Source: CAD feature listing. Evaluate the final solid. Frame: model axes, mm. A direction names the side the tool comes from. Give positions to 0.01 mm unless a question says otherwise; leave off trailing zeros. Write each loop counter-clockwise with the first axis right and the second up, starting at its lowest first coordinate (ties: lowest second). Pieces come first, ordered by that corner, then holes. Notation, with made-up numbers: M 35,-38 L 68,-38 A20 cw 68,-23 Z; hole C -25,24 d11. An arc over 180 degrees is marked long. Use CSV: the item, a comma, the result in double quotes. Start each with the question number.
from build123d import *

# Parameters (mm, degrees)
SKETCH_1_W               = 3
SKETCH_1_H               = 8
SKETCH_2_R               = 7.25
CUT_EXTRUDE_1_DEPTH      = 1
EXTRUDE_START            = 10
EXTRUDE_1_DEPTH          = 10
CUT_EXTRUDE_2_DEPTH      = 48.607194834
CUT_EXTRUDE_2_DEPTH_BACK = 48.607194834
SKETCH_4_R               = 1.55


with BuildPart() as part:
    # 草图1 → 旋转1 (revolve)
    with BuildSketch(Plane.XY, mode=Mode.PRIVATE) as revolve_1_sk:
        Polygon((0, 42), (0, 39.9), (7.85, 39.9), (15.85, 39.9), (15.85, 42), align=None)
        Polygon((0, 39.9), (0, 8), (3, 8), (7.85, 8), (7.85, 39.9), align=None)
        with Locations((1.5, 4)):
            Rectangle(SKETCH_1_W, SKETCH_1_H)
    revolve(revolve_1_sk.sketch.rotate(Axis((0, 0, 0), (0, 1, 0)), 90), axis=Axis((0, 0, 0), (0, 1, 0)))

    # 草图2 → 切除-拉伸1 (cut)
    with BuildSketch(Plane(origin=(0, 42, 0), x_dir=(1, 0, 0), z_dir=(0, 1, 0))):
        with Locations(Location((0, 0, 0), (0, 0, 270))):
            Circle(SKETCH_2_R)
    extrude(amount=-CUT_EXTRUDE_1_DEPTH, mode=Mode.SUBTRACT)

    # 草图3 → 凸台-拉伸1 (add)
    with BuildSketch(Plane(origin=(0, 41, 0), x_dir=(1, 0, 0), z_dir=(0, 1, 0)).offset(EXTRUDE_START)):
        with BuildLine():
            Line((-5.888377744, 2.752636472), (-6.707122517, 2.752636472))
            ThreePointArc((-6.707122517, 2.752636472), (-7.25, 0), (-6.707122517, -2.752636472))
            Line((-6.707122517, -2.752636472), (-5.888377744, -2.752636472))
            ThreePointArc((-5.888377744, -2.752636472), (-6.5, 0), (-5.888377744, 2.752636472))
        make_face()
        with BuildLine():
            ThreePointArc((7.25, 0), (7.11298595, 1.402829597), (6.707122517, 2.752636472))
            Line((6.707122517, 2.752636472), (5.888377744, 2.752636472))
            ThreePointArc((5.888377744, 2.752636472), (6.345252372, 1.409883801), (6.5, 0))
            ThreePointArc((6.5, 0), (6.345252372, -1.409883801), (5.888377744, -2.752636472))
            Line((5.888377744, -2.752636472), (6.707122517, -2.752636472))
            ThreePointArc((6.707122517, -2.752636472), (7.11298595, -1.402829597), (7.25, 0))
        make_face()
    extrude(amount=-EXTRUDE_1_DEPTH)

    # 草图4 → 切除-拉伸2 (cut, two sides: drawn at the far end of the back side and taken through both)
    with BuildSketch(Plane(origin=(0, 42, 0), x_dir=(1, 0, 0), z_dir=(0, 1, 0)).offset(-CUT_EXTRUDE_2_DEPTH_BACK)):
        with Locations(Location((0, -13.05, 0), (0, 0, 270))):
            Circle(SKETCH_4_R)
        with Locations(Location((-11.301631519, 6.525, 0), (0, 0, 270))):
            Circle(SKETCH_4_R)
        with Locations(Location((11.301631519, 6.525, 0), (0, 0, 270))):
            Circle(SKETCH_4_R)
    extrude(amount=CUT_EXTRUDE_2_DEPTH + CUT_EXTRUDE_2_DEPTH_BACK, mode=Mode.SUBTRACT)


solid = part.part
1. Section A-A on y = 45.5. Return loops of the section in (x, z).
2. Section B-B on x = 0. Return loops of the section in (y, z), then the cut area to 3 significant figures.
3. First-contact query: pin 1 (3 mm diameter, centred on x = 0, z = 13.05, fed in from -Y); pin 2 (8 mm diameter, centred on x = 2.5, y = 29, fed in from +Z); pin 3 (1 mm diameter, centred on x = 3.5, y = 24, fed in from -Z); pin 4 (1.5 mm diameter, centred on y = 41, z = 12, fed in from -X). Flat tips, straight axial feed; report the tip coordinate or a pass-through.
4. Pull-direction query (X, two-part tool) for faces 1 (the cylindrical face through (-6.5, 46.1, 0)), 2 (the flat face through (-7.3, 39.9, 3.3)), 3 (the cylindrical face through (-7.25, 46.56, -0.04)), 4 (the cylindrical face through (-15.715, 40.965, 2.063)); classes: released by +X, released by -X, zero draft, split by the parting line, or undercut.
5. Access query for faces 5 (the cylindrical face through (-12.815, 40.935, -6.861)), 6 (the flat face through (3.4, 8, -0.1)). Directions: +Z, -Z, +X, -X, +Y, -Y. A direction counts if a zero-diameter tool reaches every point of the face in a straight line with its end or side. Return the directions, or none.
6. Line query: probe 1 along Z at (x, y) = (3, 36); probe 2 along Y at (x, z) = (-11, 7.5); probe 3 along Z at (x, y) = (-6, 49.5). Output: solid intervals per line, ascending.
7. Section C-C on z = 13.05. Return loops of the section in (x, y), then the cut area to 3 significant figures.
8. Section D-D on y = 19. Return loops of the section in (x, z).
Resolved:
1,outline,"M -6.71,-2.75 L -5.89,-2.75 A6.5 cw -5.89,2.75 L -6.71,2.75 A7.25 ccw Z; M 5.89,-2.75 L 6.71,-2.75 A7.25 ccw 6.71,2.75 L 5.89,2.75 A6.5 cw Z"
2,outline,"M 0,-3 L 8,-3 L 8,-7.85 L 39.9,-7.85 L 39.9,-15.85 L 42,-15.85 L 42,-7.25 L 41,-7.25 L 41,7.25 L 42,7.25 L 42,11.5 L 39.9,11.5 L 39.9,7.85 L 8,7.85 L 8,3 L 0,3 Z; M 39.9,14.6 L 42,14.6 L 42,15.85 L 39.9,15.85 Z"
2,area,"594 mm2"
3,pin 1,"passes through"
3,pin 2,"stops at z = 7.85"
3,pin 3,"stops at z = -7.25"
3,pin 4,"stops at x = -11.17"
4,face 1,"undercut"
4,face 2,"zero draft"
4,face 3,"released by -X"
4,face 4,"split by the parting line"
5,face 5,"+Y, -Y"
5,face 6,"-Y"
6,probe 1,"z = -7.25 to 7.25"
6,probe 2,"y = 39.9 to 42"
6,probe 3,"z = -2.75 to -2.5, 2.5 to 2.75"
7,outline,"M -9,39.9 L -1.55,39.9 L -1.55,42 L -9,42 Z; M 1.55,39.9 L 9,39.9 L 9,42 L 1.55,42 Z"
7,area,"31.3 mm2"
8,outline,"C 0,0 d15.7"
